Can you work these out from the model? Positions are in its coordinate system, mm. A direction names the side the tool comes from. Coordinates: 2 decimals unless noted, no trailing zeros. Order: outer loops, then holes, each group sorted by start corner. A loop starts at its lowest first (then second) coordinate and runs counter-clockwise, first axis right, second up. Notation, with made-up numbers: (27.5, 83.25) -> (41.5, 83.25) arc R18 ccw to (41.5, 97.25) -> close; hole circle Ø11 at (18.25, 66.5). An arc over 180 degrees is marked (long way). Write item = value, one per line. Start each with the question number.
Autodesk Inventor part; units mm, degrees
ref_plane "Work Plane1" through (0, 0, 0) normal (0, 0, 1) x (1, 0, 0)
ref_plane "YZ Plane" through (0, 0, 0) normal (1, 0, 0) x (0, 1, 0)
ref_plane "XZ Plane" through (0, 0, 0) normal (0, 1, 0) x (-1, 0, 0)
ref_plane "Work Plane1" through (0, 0, 0) normal (0, 0, 1) x (1, 0, 0)
sketch "Sketch1" plane through (0, 0, 0) normal (0, 0, 1) x (1, 0, 0)
  circle A0 centre (0, 0) radius 2.413
  line L0 (-4.7444, -6.5405) -> (4.7444, -6.5405)
  line L1 (4.7444, -6.5405) -> (10.16, -11.9561)
  line L2 (10.16, -11.9561) -> (10.16, -16.002)
  line L3 (10.16, -16.002) -> (6.985, -16.002)
  line L4 (6.985, -16.002) -> (6.985, -15.24)
  line L5 (6.985, -15.24) -> (4.445, -15.24)
  line L6 (4.445, -15.24) -> (4.445, -19.05)
  line L7 (4.445, -19.05) -> (19.05, -19.05)
  line L8 (19.05, -19.05) -> (19.05, -4.445)
  line L9 (19.05, -4.445) -> (15.24, -4.445)
  line L10 (15.24, -4.445) -> (15.24, -6.985)
  line L11 (15.24, -6.985) -> (16.002, -6.985)
  line L12 (16.002, -6.985) -> (16.002, -10.16)
  line L13 (16.002, -10.16) -> (11.9561, -10.16)
  line L14 (11.9561, -10.16) -> (6.5405, -4.7444)
  line L15 (6.5405, -4.7444) -> (6.5405, 4.7444)
  line L16 (6.5405, 4.7444) -> (11.9561, 10.16)
  line L17 (11.9561, 10.16) -> (16.002, 10.16)
  line L18 (16.002, 10.16) -> (16.002, 6.985)
  line L19 (16.002, 6.985) -> (15.24, 6.985)
  line L20 (15.24, 6.985) -> (15.24, 4.445)
  line L21 (15.24, 4.445) -> (19.05, 4.445)
  line L22 (19.05, 4.445) -> (19.05, 19.05)
  line L23 (19.05, 19.05) -> (4.445, 19.05)
  line L24 (4.445, 19.05) -> (4.445, 15.24)
  line L25 (4.445, 15.24) -> (6.985, 15.24)
  line L26 (6.985, 15.24) -> (6.985, 16.002)
  line L27 (6.985, 16.002) -> (10.16, 16.002)
  line L28 (10.16, 16.002) -> (10.16, 11.9561)
  line L29 (10.16, 11.9561) -> (4.7444, 6.5405)
  line L30 (4.7444, 6.5405) -> (-4.7444, 6.5405)
  line L31 (-4.7444, 6.5405) -> (-10.16, 11.9561)
  line L32 (-10.16, 11.9561) -> (-10.16, 16.002)
  line L33 (-10.16, 16.002) -> (-6.985, 16.002)
  line L34 (-6.985, 16.002) -> (-6.985, 15.24)
  line L35 (-6.985, 15.24) -> (-4.445, 15.24)
  line L36 (-4.445, 15.24) -> (-4.445, 19.05)
  line L37 (-4.445, 19.05) -> (-19.05, 19.05)
  line L38 (-19.05, 19.05) -> (-19.05, 4.445)
  line L39 (-19.05, 4.445) -> (-15.24, 4.445)
  line L40 (-15.24, 4.445) -> (-15.24, 6.985)
  line L41 (-15.24, 6.985) -> (-16.002, 6.985)
  line L42 (-16.002, 6.985) -> (-16.002, 10.16)
  line L43 (-16.002, 10.16) -> (-11.9561, 10.16)
  line L44 (-11.9561, 10.16) -> (-6.5405, 4.7444)
  line L45 (-6.5405, 4.7444) -> (-6.5405, -4.7444)
  line L46 (-6.5405, -4.7444) -> (-11.9561, -10.16)
  line L47 (-11.9561, -10.16) -> (-16.002, -10.16)
  line L48 (-16.002, -10.16) -> (-16.002, -6.985)
  line L49 (-16.002, -6.985) -> (-15.24, -6.985)
  line L50 (-15.24, -6.985) -> (-15.24, -4.445)
  line L51 (-15.24, -4.445) -> (-19.05, -4.445)
  line L52 (-19.05, -4.445) -> (-19.05, -19.05)
  line L53 (-19.05, -19.05) -> (-4.445, -19.05)
  line L54 (-4.445, -19.05) -> (-4.445, -15.24)
  line L55 (-4.445, -15.24) -> (-6.985, -15.24)
  line L56 (-6.985, -15.24) -> (-6.985, -16.002)
  line L57 (-6.985, -16.002) -> (-10.16, -16.002)
  line L58 (-10.16, -16.002) -> (-10.16, -11.9561)
  line L59 (-10.16, -11.9561) -> (-4.7444, -6.5405)
  line L60 (-18.415, 19.0754) -> (-3.937, 19.0754)
  line L61 (-3.937, 19.0754) -> (-3.937, 15.2146)
  line L62 (-3.937, 15.2146) -> (3.937, 15.2146)
  line L63 (3.937, 15.2146) -> (3.937, 19.0754)
  line L64 (3.937, 19.0754) -> (18.415, 19.0754)
  line L65 (18.415, 19.0754) -> (18.415, 19.6754)
  line L66 (18.415, 19.6754) -> (-18.415, 19.6754)
  line L67 (-18.415, 19.6754) -> (-18.415, 19.0754)
  dimension "d0" = 0.635
  dimension "d1" = 0.635
  dimension "d2" = 0.0254
  dimension "d3" = 0.6
  dimension "d4" = 0.508
  dimension "d5" = 0.508
  dimension "d6" = 0.0254
extrude "Extrusion1" add sketch "Sketch1" against normal blind 83.82 contours L67 L66 L65 L64 L63 L62 L61 L60
fillet "Fillet1" radius 1.27 2 edges at (3.937, 15.2146, -41.91) (-3.937, 15.2146, -41.91)
fillet "Fillet2" radius 2.54 4 edges at (18.415, 19.3754, 0) (18.415, 19.3754, -83.82) (-18.415, 19.3754, -83.82) (-18.415, 19.3754, 0)
equation "\"d1\" = d0"
equation "\"d5\" = d4"
equation "\"d6\" = d2"
properties part number "Flat Bearing"
(1) Thinking about a two-plate mould opening in Z: for faces 4 (the face through (3.937, 18, -41)), 5 (the face through (17.651, 19.38, -0.724)), 6 (the face through (-17.691, 19.371, -83.056)), which applies, +Z half, -Z half, draft (parallel to the pull), parting line (faces both ways), or undercut?
(2) For P1, Ø7, axis at x = 13.5, z = -32.5, coming from the -Y side; P2, Ø1.3, axis at y = 17.5, z = -40.5, coming from the -X side, each with a flat end and sliding along its axis, tell me the tip position at first contact or that it passes through.
(3) Imagine slicing it at B-B (x = -8.5). Write out the boundary of the cut face in (y, z).
(4) Imagine slicing it at A-A (z = -26). Write out the boundary of the cut face in (x, y) (3 decimals).
(5) For faces 1 (the face through (11, 19.075, -41)), 2 (the face through (-3.937, 18, -41)), 3 (the face through (0, 15.215, -41)), which set-ups out of +Z, -Z, +X, -X, +Y, -Y let a thin tool reach every point of the face, with its end or its side?
(6) Imagine slicing it at C-C (y = 17.4). Write out the boundary of the cut face in (x, z), plus the area to 3 significant figures.
(7) If I drill on L1, parallel to Y at x = -7, z = -20; L2, parallel to X at y = 17.7, z = -54; L3, parallel to X at y = 15.95, z = -31, over which ranges is the centre line in solid material (lowest first)? Write a range as from..to.
Result set:
q1.face_4 = draft
q1.face_5 = +Z half
q1.face_6 = -Z half
q2.P1 = 19.08
q2.P2 = -3.94
q3.outline = (19.08, -83.82) -> (19.68, -83.82) -> (19.68, 0) -> (19.08, 0) -> close
q4.outline = (-18.415, 19.075) -> (-3.937, 19.075) -> (-3.937, 16.485) arc R1.27 ccw to (-2.667, 15.215) -> (2.667, 15.215) arc R1.27 ccw to (3.937, 16.485) -> (3.937, 19.075) -> (18.415, 19.075) -> (18.415, 19.675) -> (-18.415, 19.675) -> close
q5.face_1 = +Z, -Z, +X, -Y
q5.face_2 = +Z, -Z, -X, -Y
q5.face_3 = +Z, -Z, +X, -X, -Y
q6.outline = (-3.94, -83.82) -> (3.94, -83.82) -> (3.94, 0) -> (-3.94, 0) -> close
q6.area = 660 mm2
q7.L1 = 19.08..19.68
q7.L2 = -3.94..3.94
q7.L3 = -3.82..3.82
